```python
from build123d import *

# Parameters (mm, degrees)
SKETCH2_W                  = 125
SKETCH2_H                  = 95
SKETCH2_R                  = 28.1
SKETCH2_R_2                = 8
BOSS_EXTRUDE1_DEPTH        = 30
SKETCH10_R                 = 36.25
CUT_EXTRUDE3_DEPTH         = 12
M4X0_7_TAPPED_HOLE1_D      = 3.3
M6X1_0_TAPPED_HOLE1_D      = 5
M6X1_0_TAPPED_HOLE1_DEPTH  = 15
M6X1_0_TAPPED_HOLE1_TIP    = 1.502151548
SKETCH19_W                 = 95
SKETCH19_H                 = 30
BOSS_EXTRUDE3_DEPTH        = 2
M6X1_0_TAPPED_HOLE2_D      = 5
M6X1_0_TAPPED_HOLE2_DEPTH  = 11
M6X1_0_TAPPED_HOLE2_TIP    = 1.502151548
CIRPATTERN1_COUNT          = 2
CIRPATTERN1_ANGLE          = 45
M6X1_0_TAPPED_HOLE5_REACH  = 120.681
M6X1_0_TAPPED_HOLE5_BORE_R = 2.5
FILLET1_R                  = 2


with BuildPart() as part:
    # Sketch2 → Boss-Extrude1 (new body)
    with BuildSketch(Plane(origin=(0, 0, 0), x_dir=(1, 0, 0), z_dir=(0, 1, 0))):
        Rectangle(SKETCH2_W, SKETCH2_H)
        with Locations(Location((0, 0, 0), (0, 0, 270))):
            Circle(SKETCH2_R, mode=Mode.SUBTRACT)
        with Locations(Location((44, 29, 0), (0, 0, 270))):
            Circle(SKETCH2_R_2, mode=Mode.SUBTRACT)
        with Locations(Location((44, -29, 0), (0, 0, 270))):
            Circle(SKETCH2_R_2, mode=Mode.SUBTRACT)
        with Locations(Location((-44, -29, 0), (0, 0, 270))):
            Circle(SKETCH2_R_2, mode=Mode.SUBTRACT)
        with Locations(Location((-44, 29, 0), (0, 0, 270))):
            Circle(SKETCH2_R_2, mode=Mode.SUBTRACT)
    extrude(amount=BOSS_EXTRUDE1_DEPTH)

    # Sketch10 → Cut-Extrude3 (cut)
    with BuildSketch(Plane(origin=(0, 30, 0), x_dir=(1, 0, 0), z_dir=(0, 1, 0))):
        with Locations(Location((0, 0, 0), (0, 0, 270))):
            Circle(SKETCH10_R)
    extrude(amount=-CUT_EXTRUDE3_DEPTH, mode=Mode.SUBTRACT)

    # M4x0.7 Tapped Hole1 (through all)
    with Locations(Plane(origin=(0, 18, 0), x_dir=(1, 0, 0), z_dir=(0, 1, 0))):
        with Locations((0, 31), (31, 0), (0, -31), (-31, 0)):
            m4x0_7_tapped_hole1 = Hole(M4X0_7_TAPPED_HOLE1_D / 2)

    # M6x1.0 Tapped Hole1
    with Locations(Plane.XY.offset(47.5)):
        with Locations((-20, 15), (20, 15)):
            Hole(M6X1_0_TAPPED_HOLE1_D / 2, depth=M6X1_0_TAPPED_HOLE1_DEPTH)
            with Locations((0, 0, -(M6X1_0_TAPPED_HOLE1_DEPTH + M6X1_0_TAPPED_HOLE1_TIP / 2))):  # 118° drill point
                Cone(0, M6X1_0_TAPPED_HOLE1_D / 2, M6X1_0_TAPPED_HOLE1_TIP, mode=Mode.SUBTRACT)

    # Sketch19 → Boss-Extrude3 (add)
    with BuildSketch(Plane.ZY.offset(62.5)):
        with Locations((0, 15)):
            Rectangle(SKETCH19_W, SKETCH19_H)
    extrude(amount=BOSS_EXTRUDE3_DEPTH)

    # M6x1.0 Tapped Hole2
    with Locations(Plane(origin=(62.5, 0, 0), x_dir=(0, 0, 1), z_dir=(1, 0, 0))):
        with Locations((33, -15), (0, -15), (-33, -15)):
            Hole(M6X1_0_TAPPED_HOLE2_D / 2, depth=M6X1_0_TAPPED_HOLE2_DEPTH)
            with Locations((0, 0, -(M6X1_0_TAPPED_HOLE2_DEPTH + M6X1_0_TAPPED_HOLE2_TIP / 2))):  # 118° drill point
                Cone(0, M6X1_0_TAPPED_HOLE2_D / 2, M6X1_0_TAPPED_HOLE2_TIP, mode=Mode.SUBTRACT)

    # CirPattern1: M4x0.7 Tapped Hole1 ×2 about axis
    cirpattern1_axis = Axis((0, 0, 0), (0, -1, 0))
    for i in range(1, CIRPATTERN1_COUNT):
        add(m4x0_7_tapped_hole1.rotate(cirpattern1_axis, i * CIRPATTERN1_ANGLE / (CIRPATTERN1_COUNT - 1)), mode=Mode.SUBTRACT)

    # M6x1.0 Tapped Hole5 bore → M6x1.0 Tapped Hole5 (cut, up to next)
    with BuildSketch(Plane.XY.offset(47.5), mode=Mode.PRIVATE) as m6x1_0_tapped_hole5_sk1:
        with Locations((44, 15)):
            Circle(M6X1_0_TAPPED_HOLE5_BORE_R)
    m6x1_0_tapped_hole5_tool1 = extrude(m6x1_0_tapped_hole5_sk1.sketch, amount=-M6X1_0_TAPPED_HOLE5_REACH, mode=Mode.PRIVATE) & part.part
    # M6x1.0 Tapped Hole5 bore → M6x1.0 Tapped Hole5 (cut, up to next)
    with BuildSketch(Plane.XY.offset(47.5), mode=Mode.PRIVATE) as m6x1_0_tapped_hole5_sk2:
        with Locations((-44, 15)):
            Circle(M6X1_0_TAPPED_HOLE5_BORE_R)
    m6x1_0_tapped_hole5_tool2 = extrude(m6x1_0_tapped_hole5_sk2.sketch, amount=-M6X1_0_TAPPED_HOLE5_REACH, mode=Mode.PRIVATE) & part.part
    m6x1_0_tapped_hole5_1 = m6x1_0_tapped_hole5_tool1.solids().sort_by_distance((44, 15, 47.5))[0]
    add(m6x1_0_tapped_hole5_1, mode=Mode.SUBTRACT)
    m6x1_0_tapped_hole5_2 = m6x1_0_tapped_hole5_tool2.solids().sort_by_distance((-44, 15, 47.5))[0]
    add(m6x1_0_tapped_hole5_2, mode=Mode.SUBTRACT)
    m6x1_0_tapped_hole5 = m6x1_0_tapped_hole5_1 + m6x1_0_tapped_hole5_2  # M6x1.0 Tapped Hole5 as one shape, for the pattern or mirror that repeats it

    # Fillet1
    fillet1_edges = [part.edges().sort_by_distance(p)[0] for p in [
        (62.5, 15, 47.5),
        (62.5, 15, -47.5),
        (-64.5, 15, -47.5),
        (-64.5, 15, 47.5),
    ]]
    fillet(fillet1_edges, radius=FILLET1_R)

    # Mirror1: M6x1.0 Tapped Hole5 across plane
    add(m6x1_0_tapped_hole5.mirror(Plane.XY), mode=Mode.SUBTRACT)


solid = part.part
```
Model file for the job. Use its own axes, mm. A direction names the side the tool comes from. Give positions to 0.01 mm unless a question says otherwise; leave off trailing zeros. Write each loop counter-clockwise with the first axis right and the second up, starting at its lowest first coordinate (ties: lowest second). Pieces come first, ordered by that corner, then holes. Notation, with made-up numbers: M -33,-21.5 L 18,-21.5 A6 ccw 18,-11.5 Z; hole C 56,20.5 d8. An arc over 180 degrees is marked long. Use a Markdown table: item, result.
1) Cut at A-A (y = 24.5). List the corners of the cut face in (x, z), and give its area (3 significant figures).
Responses:
| item | result |
|---|---|
| outline | M -64.5,-45.5 A2 ccw -62.5,-47.5 L 60.5,-47.5 A2 ccw 62.5,-45.5 L 62.5,45.5 A2 ccw 60.5,47.5 L -62.5,47.5 A2 ccw -64.5,45.5 Z; hole C -44,-29 d16; hole C -44,29 d16; hole C 0,0 d72.5; hole C 44,-29 d16; hole C 44,29 d16 |
| area | 7,130 mm2 |
2) Cut at B-B (x = 11). List the corners of the cut face in (y, z), and give its area (3 significant figures).
Responses:
| item | result |
|---|---|
| outline | M 0,-47.5 L 30,-47.5 L 30,-34.54 L 18,-34.54 L 18,-25.86 L 0,-25.86 Z; M 0,25.86 L 18,25.86 L 18,34.54 L 30,34.54 L 30,47.5 L 0,47.5 Z |
| area | 1,090 mm2 |
3) Cut at C-C (x = -44). List the corners of the cut face in (y, z), and give its area (4 significant figures).
Responses:
| item | result |
|---|---|
| outline | M 0,-47.5 L 12.5,-47.5 L 12.5,-37 L 0,-37 Z; M 0,-21 L 30,-21 L 30,21 L 0,21 Z; M 0,37 L 12.5,37 L 12.5,47.5 L 0,47.5 Z; M 17.5,-47.5 L 30,-47.5 L 30,-37 L 17.5,-37 Z; M 17.5,37 L 30,37 L 30,47.5 L 17.5,47.5 Z |
| area | 1,785 mm2 |
4) Cut at D-D (z = 11). List the corners of the cut face in (x, y), and give its area (3 significant figures).
Responses:
| item | result |
|---|---|
| outline | M -64.5,0 L -25.86,0 L -25.86,18 L -34.54,18 L -34.54,30 L -64.5,30 Z; M 25.86,0 L 62.5,0 L 62.5,30 L 34.54,30 L 34.54,18 L 25.86,18 Z |
| area | 2,050 mm2 |
5) Pull direction X, two halves, no side cores. Call faces 6 (the flat face through (0, 15, 47.5)), 7 (the cylindrical face through (-41.69, 14.04, 42.13)), 8 (the flat face through (-64.5, 15, -1)): +X half, -X half, draft (parallel to the pull), parting line (faces both ways), or undercut.
Responses:
| item | result |
|---|---|
| face 6 | draft |
| face 7 | undercut |
| face 8 | -X half |
6) Tool access for faces 1 (the flat face through (0, 15, -47.5)), 2 (the cylindrical face through (56.92, 17.44, 33.54)), 3 (the cylindrical face through (46.31, 14.04, -42.13)), 4 (the cylindrical face through (-22.683, 8.874, 20.457)), 5 (the cylindrical face through (22.5, 15.1, 39.9)): list every direction of +Z, -Z, +X, -X, +Y, -Y with a clear straight run to the whole face (end or side of a thin tool).
Responses:
| item | result |
|---|---|
| face 1 | -Z, +X, -X, +Y, -Y |
| face 2 | +X |
| face 3 | -Z |
| face 4 | +Y, -Y |
| face 5 | +Z |
7) Drill centre lines: line 1 (Z direction, x = 0, y = 8.5); line 2 (X direction, y = 15, z = -39.25); line 3 (Y direction, x = 56, z = 0). Where is each one in solid material? Low to high. Write a range as from..to.
Responses:
| item | result |
|---|---|
| line 1 | z = -47.5..-32.65, -29.35..-28.1, 28.1..29.35, 32.65..47.5 |
| line 2 | x = -64.5..-46.5, -41.5..41.5, 46.5..62.5 |
| line 3 | y = 0..12.5, 17.5..30 |
8) Pin check, flat tips, straight feed: pin 1 (2 mm diameter, centred on x = -29, z = 6.5, fed in from +Y); pin 2 (3 mm diameter, centred on x = -44, y = 15, fed in from +Z); pin 3 (4 mm diameter, centred on x = 44, y = 15, fed in from +Z). Stop position of each tip, or through.
Responses:
| item | result |
|---|---|
| pin 1 | stops at y = 18 |
| pin 2 | stops at z = 21.14 |
| pin 3 | stops at z = 21.25 |
